from build123d import *

# Parameters (mm, degrees)
SKETCH6_R                        = 29
SKETCH6_R_2                      = 20
INNER_RING_DEPTH                 = 30
MOTOR_CONNECTOR_CUT_DEPTH        = 30
SKETCH9_R                        = 50
SKETCH9_R_2                      = 29
OUTSIDE_RING_EXTRUSION_DEPTH     = 30
SKETCH12_R                       = 45
SKETCH12_R_2                     = 27.5
CUT_EXTRUDE6_DEPTH               = 38
CUT_EXTRUDE6_DEPTH_BACK          = 56
SKETCH8_R                        = 2.987
MOTOR_CONNECTOR_HOLES_DEPTH      = 27
MOTOR_CONNECTOR_HOLES_DEPTH_BACK = 41
SKETCH10_R                       = 27.404299948
PATTERN_DEPTH                    = 30
SKETCH13_R                       = 45
SKETCH13_R_2                     = 40
BOSS_EXTRUDE1_DEPTH              = 30
CUT_EXTRUDE7_DEPTH               = 13
CUT_EXTRUDE8_DEPTH               = 15
CUT_EXTRUDE9_DEPTH               = 17
CUT_EXTRUDE10_DEPTH              = 17


with BuildPart() as part:
    # Sketch6 → Inner Ring (new body)
    with BuildSketch(Plane.XY):
        Circle(SKETCH6_R)
        Circle(SKETCH6_R_2, mode=Mode.SUBTRACT)
    extrude(amount=-INNER_RING_DEPTH)

    # Sketch7 → Motor Connector Cut (add)
    with BuildSketch(Plane.XY):
        with BuildLine():
            ThreePointArc((20, 0), (19.840593925, 2.52008585), (19.364916731, 5))
            Line((19.364916731, 5), (9.999996731, 5))
            Line((9.999996731, 5), (9.999996731, -5))
            Line((9.999996731, -5), (19.364916731, -5))
            ThreePointArc((19.364916731, -5), (19.840593925, -2.52008585), (20, 0))
        make_face()
        with BuildLine():
            ThreePointArc((5, 19.364916731), (0, 20), (-5, 19.364916731))
            Line((-5, 19.364916731), (-5, 9.999996731))
            Line((-5, 9.999996731), (5, 9.999996731))
            Line((5, 9.999996731), (5, 19.364916731))
        make_face()
        with BuildLine():
            Line((-9.999996731, -5), (-9.999996731, 5))
            Line((-9.999996731, 5), (-19.364916731, 5))
            ThreePointArc((-19.364916731, 5), (-20, 0), (-19.364916731, -5))
            Line((-19.364916731, -5), (-9.999996731, -5))
        make_face()
        with BuildLine():
            Line((-5, -9.999996731), (-5, -19.364916731))
            ThreePointArc((-5, -19.364916731), (0, -20), (5, -19.364916731))
            Line((5, -19.364916731), (5, -9.999996731))
            Line((5, -9.999996731), (-5, -9.999996731))
        make_face()
    extrude(amount=-MOTOR_CONNECTOR_CUT_DEPTH)

    # Sketch9 → Outside Ring Extrusion (add)
    with BuildSketch(Plane.XY):
        Circle(SKETCH9_R)
        Circle(SKETCH9_R_2, mode=Mode.SUBTRACT)
    extrude(amount=-OUTSIDE_RING_EXTRUSION_DEPTH)

    # Sketch12 → Cut-Extrude6 (cut, two sides)
    with BuildSketch(Plane.XY) as cut_extrude6_sk:
        Circle(SKETCH12_R)
        Circle(SKETCH12_R_2, mode=Mode.SUBTRACT)
    extrude(amount=CUT_EXTRUDE6_DEPTH, mode=Mode.SUBTRACT)
    extrude(cut_extrude6_sk.sketch, amount=-CUT_EXTRUDE6_DEPTH_BACK, mode=Mode.SUBTRACT)

    # Sketch8 → Motor Connector Holes (cut, two sides)
    with BuildSketch(Plane.XY) as motor_connector_holes_sk:
        with Locations((0, 17.75)):
            Circle(SKETCH8_R)
        with Locations((17.75, 0)):
            Circle(SKETCH8_R)
        with Locations((0, -17.75)):
            Circle(SKETCH8_R)
        with Locations((-17.75, 0)):
            Circle(SKETCH8_R)
    extrude(amount=MOTOR_CONNECTOR_HOLES_DEPTH, mode=Mode.SUBTRACT)
    extrude(motor_connector_holes_sk.sketch, amount=-MOTOR_CONNECTOR_HOLES_DEPTH_BACK, mode=Mode.SUBTRACT)

    # Sketch10 → Pattern (add)
    with BuildSketch(Plane.XY):
        with BuildLine():
            ThreePointArc((24.317625284, 15.800414568), (34.856582319, 15.291767932), (43.817916626, 9.721954269))
            ThreePointArc((43.817916626, 9.721954269), (41.607188912, 16.793289988), (38.263814419, 23.404867172))
            ThreePointArc((38.263814419, 23.404867172), (32.064348025, 25.470287935), (25.530148518, 25.530148518))
            ThreePointArc((25.530148518, 25.530148518), (25.475284033, 32.034279432), (23.432821057, 38.209639668))
            ThreePointArc((23.432821057, 38.209639668), (20.212556871, 40.002288656), (16.856128399, 41.524812789))
            ThreePointArc((16.856128399, 41.524812789), (13.384732217, 42.767397097), (9.823095744, 43.720997037))
            ThreePointArc((9.823095744, 43.720997037), (15.312499865, 34.789679765), (15.800414568, 24.317625284))
            ThreePointArc((15.800414568, 24.317625284), (0, 29), (-15.800414568, 24.317625284))
            ThreePointArc((-15.800414568, 24.317625284), (-15.312499865, 34.789679765), (-9.823095744, 43.720997037))
            ThreePointArc((-9.823095744, 43.720997037), (-16.854754984, 41.52536899), (-23.432821057, 38.209639668))
            ThreePointArc((-23.432821057, 38.209639668), (-25.475284033, 32.034279432), (-25.530148518, 25.530148518))
            ThreePointArc((-25.530148518, 25.530148518), (-32.064348025, 25.470287935), (-38.263814419, 23.404867172))
            ThreePointArc((-38.263814419, 23.404867172), (-41.607188912, 16.793289988), (-43.817916626, 9.721954269))
            ThreePointArc((-43.817916626, 9.721954269), (-34.856582319, 15.291767932), (-24.317625284, 15.800414568))
            ThreePointArc((-24.317625284, 15.800414568), (-29, 0), (-24.317625284, -15.800414568))
            ThreePointArc((-24.317625284, -15.800414568), (-34.894848495, -15.279799844), (-43.87309253, -9.663767027))
            ThreePointArc((-43.87309253, -9.663767027), (-41.716263612, -16.713446711), (-38.435015504, -23.315212041))
            ThreePointArc((-38.435015504, -23.315212041), (-32.159621016, -25.454161245), (-25.530148518, -25.530148518))
            ThreePointArc((-25.530148518, -25.530148518), (-25.448803812, -32.190695038), (-23.285614603, -38.490703716))
            ThreePointArc((-23.285614603, -38.490703716), (-16.649731385, -41.799208281), (-9.559859326, -43.970581744))
            ThreePointArc((-9.559859326, -43.970581744), (-15.258354287, -34.962784804), (-15.800414568, -24.317625284))
            ThreePointArc((-15.800414568, -24.317625284), (0, -29), (15.800414568, -24.317625284))
            ThreePointArc((15.800414568, -24.317625284), (15.258354287, -34.962784804), (9.559859326, -43.970581744))
            ThreePointArc((9.559859326, -43.970581744), (16.649731385, -41.799208281), (23.285614603, -38.490703716))
            ThreePointArc((23.285614603, -38.490703716), (25.448803812, -32.190695038), (25.530148518, -25.530148518))
            ThreePointArc((25.530148518, -25.530148518), (32.159621016, -25.454161245), (38.435015504, -23.315212041))
            ThreePointArc((38.435015504, -23.315212041), (41.716263612, -16.713446711), (43.87309253, -9.663767027))
            ThreePointArc((43.87309253, -9.663767027), (34.894848495, -15.279799844), (24.317625284, -15.800414568))
            ThreePointArc((24.317625284, -15.800414568), (29, 0), (24.317625284, 15.800414568))
        make_face()
        with Locations((-0.095700052, 0)):
            Circle(SKETCH10_R, mode=Mode.SUBTRACT)
    extrude(amount=-PATTERN_DEPTH)

    # Sketch13 → Boss-Extrude1 (add)
    with BuildSketch(Plane.XY):
        Circle(SKETCH13_R)
        Circle(SKETCH13_R_2, mode=Mode.SUBTRACT)
    extrude(amount=-BOSS_EXTRUDE1_DEPTH)

    # Sketch14 → Cut-Extrude7 (cut)
    with BuildSketch(Plane(origin=(0, 50, 0), x_dir=(1, 0, 0), z_dir=(0, 1, 0))):
        with BuildLine():
            ThreePointArc((0, 16.5), (-1.5, 15), (0, 13.5))
            Line((0, 13.5), (0, 16.5))
        make_face()
        with BuildLine():
            Line((0, 16.5), (0, 13.5))
            ThreePointArc((0, 13.5), (1.060660172, 13.939339828), (1.5, 15))
            ThreePointArc((1.5, 15), (1.060660172, 16.060660172), (0, 16.5))
        make_face()
    extrude(amount=-CUT_EXTRUDE7_DEPTH, mode=Mode.SUBTRACT)

    # Sketch15 → Cut-Extrude8 (cut)
    with BuildSketch(Plane(origin=(0, -50, 0), x_dir=(1, 0, 0), z_dir=(0, 1, 0))):
        with BuildLine():
            ThreePointArc((0, 16.5), (-1.5, 15), (0, 13.5))
            Line((0, 13.5), (0, 16.5))
        make_face()
        with BuildLine():
            Line((0, 16.5), (0, 13.5))
            ThreePointArc((0, 13.5), (1.060660172, 13.939339828), (1.5, 15))
            ThreePointArc((1.5, 15), (1.060660172, 16.060660172), (0, 16.5))
        make_face()
    extrude(amount=CUT_EXTRUDE8_DEPTH, mode=Mode.SUBTRACT)

    # Sketch16 → Cut-Extrude9 (cut)
    with BuildSketch(Plane(origin=(-50, 0, 0), x_dir=(0, 0, -1), z_dir=(1, 0, 0))):
        with BuildLine():
            ThreePointArc((16.5, 0), (15, 1.5), (13.5, 0))
            Line((13.5, 0), (16.5, 0))
        make_face()
        with BuildLine():
            Line((16.5, 0), (13.5, 0))
            ThreePointArc((13.5, 0), (15, -1.5), (16.5, 0))
        make_face()
    extrude(amount=CUT_EXTRUDE9_DEPTH, mode=Mode.SUBTRACT)

    # Sketch17 → Cut-Extrude10 (cut)
    with BuildSketch(Plane(origin=(50, 0, 0), x_dir=(0, 0, -1), z_dir=(1, 0, 0))):
        with BuildLine():
            ThreePointArc((16.5, 0), (15, 1.5), (13.5, 0))
            Line((13.5, 0), (16.5, 0))
        make_face()
        with BuildLine():
            Line((16.5, 0), (13.5, 0))
            ThreePointArc((13.5, 0), (15, -1.5), (16.5, 0))
        make_face()
    extrude(amount=-CUT_EXTRUDE10_DEPTH, mode=Mode.SUBTRACT)


solid = part.part
The model under review builds one solid part; all positions refer to its coordinate system, in mm. A direction names the side the tool comes from. Give positions to 0.01 mm unless a question says otherwise; leave off trailing zeros. Write each loop counter-clockwise with the first axis right and the second up, starting at its lowest first coordinate (ties: lowest second). Pieces come first, ordered by that corner, then holes.
1. Add section D-D, the plane z = -5. Count the separate pieces of the cut face and the enclosed holes in it, plus the area to 3 significant figures.
2. Wall thickness on L1, parallel to Y at x = 0, z = -14.5; L2, parallel to Y at x = 0, z = -21.5; L3, parallel to X at y = 30, z = -15.5: over which ranges is each line inside the solid? List them lowest first.
3. Tool access review of faces 3 (the flat face through (-15, -5, -15)), 4 (the cylindrical face through (-45.06, -0.07, -16.5)): name each direction out of +Z, -Z, +X, -X, +Y, -Y from which nothing blocks a thin tool from reaching the whole face with its end or side.
4. Add section A-A, the plane y = 17.75. Write out the cut boundary in (x, z), plus the area to 3 significant figures.
5. Draft analysis for pull direction X (two halves, no side actions). For faces 1 (the flat face through (-0.7, -10.4, -30)), 2 (the flat face through (-10, 0, -15)), state which applies: +X half, -X half, draft (parallel to the pull), parting line (faces both ways), or undercut.
6. For P1, Ø10.5, axis at y = 14, z = -21.5, coming from the +X side; P2, Ø12, axis at x = -13.5, z = -3.5, coming from the -Y side; P3, Ø1, axis at x = -32.5, z = -4.5, coming from the -Y side; P4, Ø8, axis at x = 0, y = -17.75, coming from the +Z side, all flat-tipped, find the tip position at first contact; note any pin that passes through.
7. Add section C-C, the plane y = 42. Write out the cut boundary in (x, z).
Worked answers:
1. separate pieces: 1
1. enclosed holes: 13
1. area: 5,380 mm2
2. L1: y = -29 to -20.74, -14.76 to -10, 10 to 14.76, 20.74 to 29
2. L2: y = -50 to -40, -29 to -20.74, -14.76 to -10, 10 to 14.76, 20.74 to 29, 40 to 50
2. L3: x = -40 to -26.46, -25.71 to -16.2, 16.2 to 25.71, 26.46 to 40
3. face 3: +Z, -Z
3. face 4: -X
4. outline: (-46.74, -30) - (-9.22, -30) - (-9.22, 0) - (-46.74, 0) - close; (-5, -30) - (-2.99, -30) - (-2.99, 0) - (-5, 0) - close; (2.99, -30) - (5, -30) - (5, 0) - (2.99, 0) - close; (9.22, -30) - (46.74, -30) - (46.74, 0) - (9.22, 0) - close
4. area: 2,370 mm2
5. face 1: draft
5. face 2: undercut
6. P1: stops at x = 49.23
6. P2: stops at y = -49.43
6. P3: stops at y = -38.42
6. P4: stops at z = 0
7. outline: (-27.13, -30) - (27.13, -30) - (27.13, 0) - (-27.13, 0) - close; hole circle Ø3 at (0, -15)
